Could you check a few things on this model? Use its own coordinates, in mm. Round coordinates to 2 decimals unless told otherwise and drop trailing zeros. Write each loop counter-clockwise with the first axis right and the second up, starting at its lowest first coordinate (ties: lowest second). Pieces come first, ordered by that corner, then holes. Notation, with made-up numbers: (22.5, -22) -> (57.5, -22) arc R6 ccw to (57.5, -11) -> close; hole circle Ø6 at (60.5, 36.5). An arc over 180 degrees is marked (long way). Answer in a Markdown table with one row per item.
from build123d import *

# Parameters (mm, degrees)
F1_DEPTH = 1.27
F2_SIZE2 = 1.524
F2_SIZE  = 0.635
F3_SIZE2 = 0.63499
F3_SIZE  = 1.52399


# Not quite as in the source:
# - a fillet or chamfer is up to 0.001 mm smaller than in the source, because OpenCascade refuses the exact size


with BuildPart() as f1:
    # F0 (on Top) → F1 (new body)
    with BuildSketch(Plane.XY):
        with BuildLine():
            Line((-36.8330654015, 25.4), (-36.8330654015, 0))
            Line((-36.8330654015, 0), (-31.7530654015, 0))
            Line((-31.7530654015, 0), (-31.7530654015, 25.4))
            Line((-31.7530654015, 25.4), (-31.7530654015, 38.1))
            Line((-31.7530654015, 38.1), (-29.6483766288, 55.6414723396))
            ThreePointArc((-29.6483766288, 55.6414723396), (-30.8576350362, 66.7535648315), (-36.8330654015, 76.2))
            Line((-36.8330654015, 76.2), (-36.8330654015, 25.4))
        make_face()
    extrude(amount=F1_DEPTH)

    # F2
    f2_edges = [f1.edges().sort_by_distance(p)[0] for p in [
        (-30.857635, 66.753565, 0),
    ]]
    f2_side = f1.faces().sort_by_distance((-30.857635, 66.753565, 0.635))[0]
    chamfer(f2_edges, length=F2_SIZE, length2=F2_SIZE2, reference=f2_side)

    # F3 (size 1.524 and 0.635 in the source; OpenCascade refuses exactly that, so slightly less here)
    f3_edges = [f1.edges().sort_by_distance(p)[0] for p in [
        (-30.857635, 66.753565, 1.27),
    ]]
    f3_side = f1.faces().sort_by_distance((-33.993145, 38.475909, 1.27))[0]
    chamfer(f3_edges, length=F3_SIZE, length2=F3_SIZE2, reference=f3_side)


solid = f1.part
1) Please list where these lines run through material, in increasing order: line 1 (X direction, y = 27, z = 0.8); line 2 (Z direction, x = -31, y = 58); line 3 (Z direction, x = -30.25, y = 63).
Findings:
| item | result |
|---|---|
| line 1 | x = -36.83 to -31.75 |
| line 2 | z = 0 to 1.27 |
| line 3 | z = 0.48 to 0.79 |
2) Imagine slicing it at A-A, the plane y = 37. Please give me the cut outline in (x, z).
Findings:
| item | result |
|---|---|
| outline | (-36.83, 0) -> (-31.75, 0) -> (-31.75, 1.27) -> (-36.83, 1.27) -> close |
3) Imagine slicing it at B-B, the plane z = 0.35. Please give me the cut outline in (x, y), plus the area to 3 significant figures.
Findings:
| item | result |
|---|---|
| outline | (-36.83, 0) -> (-31.75, 0) -> (-31.75, 43.84) -> (-30.33, 55.72) arc R24.06 ccw to (-36.83, 75.23) -> close |
| area | 387 mm^2 |
